The model under review builds one solid part; all positions refer to its coordinate system, in mm. Face numbers are marked on the shaded views. A direction names the side the tool comes from. Coordinates: 2 decimals unless noted, no trailing zeros. Loops run counter-clockwise (first coordinate to the right, second up) from the corner with the lowest first, then second, coordinate; pieces in that order, holes last. Notation, with made-up numbers: (14.5, -19) - (49.5, -19) arc R14 cw to (49.5, -15) - close; hole circle Ø10 at (-21, 76). An arc over 180 degrees is marked (long way). Answer in a Markdown table with one row per item. Add a question column.
(1) We need section D-D on z = 13.25. Write out the cut boundary in (x, y).
(2) Mouldability with a two-part tool opening along X and no side actions: class the marked faces 1, 2 and 3 as +X half, -X half, draft (parallel to the pull), parting line (faces both ways), or undercut.
(3) We need section C-C on x = 69. Write out the cut boundary in (y, z).
(4) We need section A-A on z = 6.25. Write out the cut boundary in (x, y), plus the area to 3 significant figures.
(5) We need section B-B on y = -30. Write out the cut boundary in (x, z).
(6) For line 1 along X through (y, z) = (35.75, 7.5); line 2 along Y through (x, z) = (42.5, 6.25); line 3 along X through (y, z) = (17, 3.75), list the stretches that pass through material, from the lowest coordinate up.
(7) Machinability: for the marked faces 4, 5, 6, 7 and 8, which of the approach directions +Z, -Z, +X, -X, +Y, -Y give a long, thin tool a straight path to every point of the face, cutting with its end or side? Answer none if there is none.
(8) For P1, Ø5, axis at x = 46.2, y = -28.62, coming from the +Z side; P2, Ø6, axis at x = 20, y = -18, coming from the -Z side; P3, Ø6, axis at x = 68.7, z = 7.5, coming from the -Y side; P4, Ø8, axis at y = -24.5, z = 12, coming from the -X side, all flat-tipped, find the tip position at first contact; note any pin that passes through.
from build123d import *

# Parameters (mm, degrees)
SKETCH_1_R          = 12
SKETCH_1_R_2        = 4.25
EXTRUDE_1_DEPTH     = 15
SKETCH_2_R          = 13.05
CUT_EXTRUDE_1_DEPTH = 10
SKETCH_3_R          = 2.6
CUT_EXTRUDE_2_DEPTH = 81
SKETCH_5_R          = 2.6
CUT_EXTRUDE_3_DEPTH = 10


with BuildPart() as part:
    # 草图1 → 凸台-拉伸1 (new body)
    with BuildSketch(Plane.XY):
        Polygon((-33.800989673, 26.383498279), (-27.44059998, 26.383498279), (-18.800989673, 26.383498279), (-18.800989673, 10.67282016), (30.488332208, -38.616501721), (61.199010327, -38.616501721), (61.199010327, 26.383498279), (76.199010327, 26.383498279), (76.199010327, 41.383498279), (56.199010327, 41.383498279), (-33.800989673, 41.383498279), align=None)
        with Locations((41.199010327, 21.383498279)):
            Circle(SKETCH_1_R, mode=Mode.SUBTRACT)
        with Locations((46.199010327, -28.616501721)):
            Circle(SKETCH_1_R_2, mode=Mode.SUBTRACT)
        with BuildLine():
            Line((-11.126891481, 11.484003342), (3.015244143, 25.626138966))
            ThreePointArc((3.015244143, 25.626138966), (10.086311955, 25.626138966), (10.086311955, 18.555071154))
            Line((10.086311955, 18.555071154), (-4.055823669, 4.41293553))
            Line((-4.055823669, 4.41293553), (-11.126891481, 11.484003342))
        make_face(mode=Mode.SUBTRACT)
    extrude(amount=EXTRUDE_1_DEPTH)

    # 草图2 → 切除-拉伸1 (cut)
    with BuildSketch(Plane(origin=(0, 0, 15), x_dir=(-1, 0, 0), z_dir=(0, 0, -1))):
        with Locations((-41.199010327, 21.383498279)):
            Circle(SKETCH_2_R)
    extrude(amount=CUT_EXTRUDE_1_DEPTH, mode=Mode.SUBTRACT)

    # 草图3 → 切除-拉伸2 (cut, through all)
    with BuildSketch(Plane(origin=(0, 41.383498279, 0), x_dir=(1, 0, 0), z_dir=(0, 1, 0))):
        with Locations((-26.300989673, -7.5)):
            Circle(SKETCH_3_R)
        with Locations((68.699010327, -7.5)):
            Circle(SKETCH_3_R)
    extrude(amount=-CUT_EXTRUDE_2_DEPTH, mode=Mode.SUBTRACT)

    # 草图5 → 切除-拉伸3 (cut)
    with BuildSketch(Plane(origin=(-4.064084756, -4.064084756, 0), x_dir=(0, 0, 1), z_dir=(-0.707106781, -0.707106781, 0))):
        with Locations((7.5, 10.9911308)):
            Circle(SKETCH_5_R)
    extrude(amount=-CUT_EXTRUDE_3_DEPTH, mode=Mode.SUBTRACT)


solid = part.part
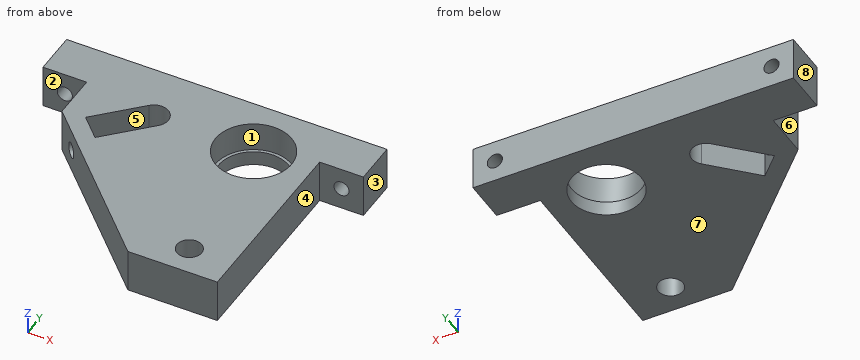
Outcome:
| question | item | result |
|---|---|---|
| 1 | outline | (-33.8, 26.38) - (-18.8, 26.38) - (-18.8, 10.67) - (30.49, -38.62) - (61.2, -38.62) - (61.2, 26.38) - (76.2, 26.38) - (76.2, 41.38) - (-33.8, 41.38) - close; hole (-11.13, 11.48) - (-4.06, 4.41) - (10.09, 18.56) arc R5 ccw to (3.02, 25.63) - close; hole circle Ø26.1 at (41.2, 21.38); hole circle Ø8.5 at (46.2, -28.62) |
| 2 | face 1 | undercut |
| 2 | face 2 | draft |
| 2 | face 3 | +X half |
| 3 | outline | (26.38, 0) - (41.38, 0) - (41.38, 4.92) - (26.38, 4.92) - close; (26.38, 10.08) - (41.38, 10.08) - (41.38, 15) - (26.38, 15) - close |
| 4 | outline | (-33.8, 26.38) - (-28.58, 26.38) - (-28.58, 41.38) - (-33.8, 41.38) - close; (-24.02, 26.38) - (-18.8, 26.38) - (-18.8, 10.67) - (-13.45, 5.32) - (-9.21, 9.56) - (-11.13, 11.48) - (3.02, 25.63) arc R5 cw to (10.09, 18.56) - (-4.06, 4.41) - (-5.98, 6.34) - (-10.22, 2.1) - (30.49, -38.62) - (61.2, -38.62) - (61.2, 26.38) - (66.42, 26.38) - (66.42, 41.38) - (-24.02, 41.38) - close; (70.98, 26.38) - (76.2, 26.38) - (76.2, 41.38) - (70.98, 41.38) - close; hole circle Ø26.1 at (41.2, 21.38); hole circle Ø8.5 at (46.2, -28.62) |
| 4 | area | 4,640 mm² |
| 5 | outline | (21.87, 0) - (42.18, 0) - (42.18, 15) - (21.87, 15) - close; (50.22, 0) - (61.2, 0) - (61.2, 15) - (50.22, 15) - close |
| 6 | line 1 | -33.8 to -28.9, -23.7 to 66.1, 71.3 to 76.2 |
| 6 | line 2 | -38.62 to -30.71, -26.52 to 8.4, 34.37 to 41.38 |
| 6 | line 3 | -18.8 to -5.61, 8.53 to 30.03, 52.37 to 61.2 |
| 7 | face 4 | +Z, -Z, +X, -Y |
| 7 | face 5 | +Z, -Z |
| 7 | face 6 | +Z, -Z, -X, -Y |
| 7 | face 7 | -Z, +X, -X, +Y, -Y |
| 7 | face 8 | +Z, -Z, -X, +Y, -Y |
| 8 | P1 | through |
| 8 | P2 | z = 0 |
| 8 | P3 | y = 26.38 |
| 8 | P4 | x = 12.37 |
